from build123d import *

# Parameters (mm, degrees)
ESQUISSE1_W             = 80
ESQUISSE1_H             = 80
EXTRUSION1_DEPTH        = 1
CONG_1_R                = 5
ESQUISSE3_R             = 4
ENL_V_MAT_EXTRU_1_DEPTH = 2
ESQUISSE4_W             = 8
ESQUISSE4_H             = 8
ENL_V_MAT_EXTRU_2_DEPTH = 2


with BuildPart() as part:
    # Esquisse1 → Extrusion1 (new body)
    with BuildSketch(Plane(origin=(0, 0, 0), x_dir=(1, 0, 0), z_dir=(0, 1, 0))):
        with Locations((40, 40)):
            Rectangle(ESQUISSE1_W, ESQUISSE1_H)
    extrude(amount=EXTRUSION1_DEPTH)

    # Congé1
    cong_1_edges = [part.edges().sort_by_distance(p)[0] for p in [
        (0, 0.5, -80),
        (80, 0.5, -80),
        (80, 0.5, 0),
        (0, 0.5, 0),
    ]]
    fillet(cong_1_edges, radius=CONG_1_R)

    # Esquisse3 → Enlèv. mat.-Extru.1 (cut, through all)
    with BuildSketch(Plane(origin=(0, 1, 0), x_dir=(1, 0, 0), z_dir=(0, 1, 0))):
        with Locations((40, 40)):
            Circle(ESQUISSE3_R)
    extrude(amount=-ENL_V_MAT_EXTRU_1_DEPTH, mode=Mode.SUBTRACT)

    # Esquisse4 → Enlèv. mat.-Extru.2 (cut, through all)
    with BuildSketch(Plane(origin=(0, 1, 0), x_dir=(1, 0, 0), z_dir=(0, 1, 0))):
        with Locations((7.5, 40)):
            Rectangle(ESQUISSE4_W, ESQUISSE4_H)
    extrude(amount=-ENL_V_MAT_EXTRU_2_DEPTH, mode=Mode.SUBTRACT)


solid = part.part
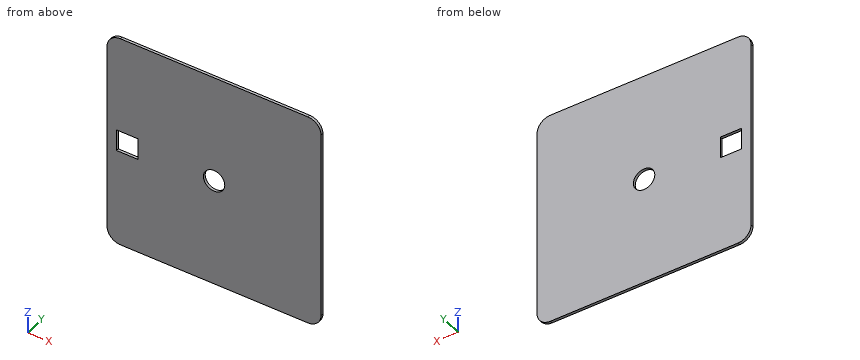
Input: part model. Units: mm. Frame: model coordinates. Give positions to 0.01 mm unless a question says otherwise; leave off trailing zeros. Loops run counter-clockwise (first coordinate to the right, second up) from the corner with the lowest first, then second, coordinate; pieces in that order, holes last. Notation, with made-up numbers: M 48,-39.5 L 88,-39.5 A19 cw 88,-12.5 Z; hole C 66.5,62 d7. An arc over 180 degrees is marked long. Use CSV: the item, a comma, the result in double quotes.
(1) Section B-B, the plane z = -40. Return loops of the section in (x, y).
Outcome:
outline,"M 0,0 L 3.5,0 L 3.5,1 L 0,1 Z; M 11.5,0 L 36,0 L 36,1 L 11.5,1 Z; M 44,0 L 80,0 L 80,1 L 44,1 Z"
(2) Material intervals for L1, parallel to X at y = 0.65, z = -40; L2, parallel to Z at x = 40, y = 0.75; L3, parallel to X at y = 0.7, z = -37, sorted ascending. Write a range as [from, to].
Outcome:
L1,"x = [0, 3.5], [11.5, 36], [44, 80]"
L2,"z = [-80, -44], [-36, 0]"
L3,"x = [0, 3.5], [11.5, 37.35], [42.65, 80]"
(3) Section A-A, the plane x = 40. Return loops of the section in (y, z).
Outcome:
outline,"M 0,-80 L 1,-80 L 1,-44 L 0,-44 Z; M 0,-36 L 1,-36 L 1,0 L 0,0 Z"
(4) Section C-C, the plane y = 0.5. Return loops of the section in (x, z).
Outcome:
outline,"M 0,-75 A5 ccw 5,-80 L 75,-80 A5 ccw 80,-75 L 80,-5 A5 ccw 75,0 L 5,0 A5 ccw 0,-5 Z; hole M 3.5,-44 L 11.5,-44 L 11.5,-36 L 3.5,-36 Z; hole C 40,-40 d8"
